```python
from build123d import *

# Parameters (mm, degrees)
F0_R     = 3.81
F4_DEPTH = 12.7


with BuildPart() as f2:
    # F2: sweep along a path in F1
    with BuildLine(Plane.XZ) as f2_path:
        ThreePointArc((25.4, 25.4), (7.439488, 17.960512), (0, 0))
    # F0 (on Top) → F2 (sweep)
    with BuildSketch(Plane.XY):
        Circle(F0_R)
    sweep(path=f2_path.line)

    # F3: sweep along a path in F1
    with BuildLine(Plane.XZ) as f3_path:
        ThreePointArc((0, 0), (-7.439488, 17.960512), (-25.4, 25.4))
    # F0 (on Top) → F3 (sweep)
    with BuildSketch(Plane.XY):
        Circle(F0_R)
    sweep(path=f3_path.line)

    # F2_face (on face) → F4 (join)
    with BuildSketch(Plane(origin=(0, 0, 0), x_dir=(1, 0, 0), z_dir=(0, 0, -1))):
        with BuildLine():
            ThreePointArc((0, -3.81), (2.694077, -2.694077), (3.81, 0))
            ThreePointArc((3.81, 0), (2.694077, 2.694077), (0, 3.81))
            ThreePointArc((0, 3.81), (-3.81, 0), (0, -3.81))
        make_face()
    extrude(amount=F4_DEPTH)


solid = f2.part
```
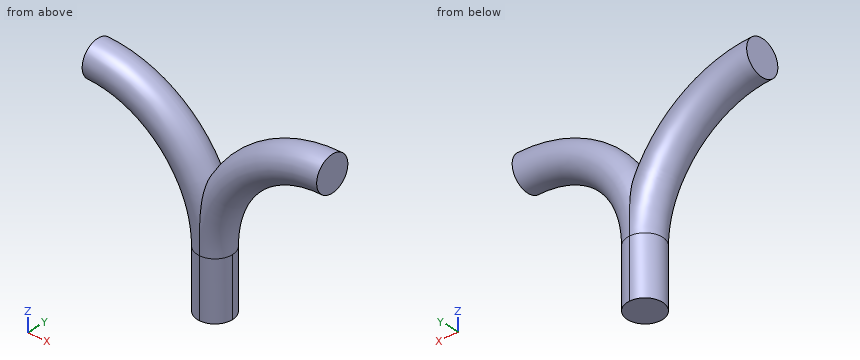
Verification items for the finished model (mm, model axes). Coordinates: 2 decimals unless noted, no trailing zeros. Loops run counter-clockwise (first coordinate to the right, second up) from the corner with the lowest first, then second, coordinate; pieces in that order, holes last. Notation, with made-up numbers: (17.25, -37) - (61.25, -37) arc R21 ccw to (61.25, 2) - close; hole circle Ø10 at (62, -16). An arc over 180 degrees is marked (long way). Answer as a JSON object with one key per item and string values.
(1) Cross-section at B-B, the plane z = -7. Record the boundary of the cut face in (x, y).
Response:
{"outline": "circle Ø7.62 at (0, 0)"}
(2) Go/stop test with flat-tipped pins: pin 1 Ø12 at (x, z) = (8.5, 4.5) entering from +Y; pin 2 Ø2 at (x, y) = (-12, -1.5) entering from +Z; pin 3 Ø2 at (y, z) = (-2, 13.5) entering from +X. Record where each tip stops, or that it passes through.
Response:
{"pin 1": "stops at y = 3.3", "pin 2": "stops at z = 26.24", "pin 3": "stops at x = 8.87"}
(3) Cross-section at C-C, the plane y = -2.5. Record the boundary of the cut face in (x, z), then the cut area to 3 significant figures.
Response:
{"outline": "(-25.4, 22.52) arc R22.52 cw to (-2.88, 0) - (-2.88, -12.7) - (2.88, -12.7) - (2.88, 0) arc R22.52 cw to (25.4, 22.52) - (25.4, 28.28) arc R28.28 ccw to (0, 12.42) arc R28.28 ccw to (-25.4, 28.28) - close", "area": "484 mm²"}
(4) Cross-section at A-A, the plane y = 1.75. Record the boundary of the cut face in (x, z).
Response:
{"outline": "(-25.4, 22.02) arc R22.02 cw to (-3.38, 0) - (-3.38, -12.7) - (3.38, -12.7) - (3.38, 0) arc R22.02 cw to (25.4, 22.02) - (25.4, 28.78) arc R28.78 ccw to (0, 13.54) arc R28.78 ccw to (-25.4, 28.78) - close"}
(5) Scan lines: line 1 along X through (y, z) = (-0.25, 24); line 2 along X through (y, z) = (-0.25, -4.5); line 3 along X through (y, z) = (-1.75, 19). Record each from-to range of solid material in increasing order.
Response:
{"line 1": "x = -25.4 to -8.76, 8.76 to 25.4", "line 2": "x = -3.8 to 3.8", "line 3": "x = -14.28 to -3.78, 3.78 to 14.28"}
